Check sheet for the modelled part. Datum: model origin and axes. Units: mm. A direction names the side the tool comes from. Round coordinates to 2 decimals unless told otherwise and drop trailing zeros. Order: outer loops, then holes, each group sorted by start corner. A loop starts at its lowest first (then second) coordinate and runs counter-clockwise, first axis right, second up.
Q1. Mould release check, pull along Z, two halves, no side actions. Record for faces 5 (the flat face through (7, 5, -70)), 6 (the flat face through (118, 20, -120)), 7 (the flat face through (13, 10, -2)): +Z half, -Z half, draft (parallel to the pull), parting line (faces both ways), or undercut.
Q2. Cross-section at D-D on y = 14. Record the cut outline in (x, z), then the cut area to 3 significant figures.
Q3. Scan lines: probe 1 along X at (y, z) = (14, 90); probe 2 along Z at (x, y) = (40, 27.5); probe 3 along Y at (x, z) = (46.5, 36). Record each from-to range of solid material in increasing order.
Q4. Cross-section at B-B on z = 45. Record the cut outline in (x, y), then the cut area to 3 significant figures.
Q5. Depth check by flat-ended pin: P1, Ø8, axis at x = 230.5, z = 47, coming from the +Y side; P2, Ø10, axis at y = 21, z = 48.5, coming from the -X side; P3, Ø5, axis at y = 34.5, z = 90, coming from the +X side. Enter the tip coordinate at first touch or a pass-through.
Q6. Cross-section at C-C on y = 31. Record the cut outline in (x, z), then the cut area to 3 significant figures.
Q7. Cross-section at A-A on x = 78. Record the cut outline in (y, z), then the cut area to 3 significant figures.
Q8. Set-up check for faces 1 (the flat face through (118.687, 32.395, 69.932)), 2 (the flat face through (233, 5, 70)), 3 (the flat face through (227, 10, -2)), 4 (the flat face through (26.245, 22, 2)): record each of +Z, -Z, +X, -X, +Y, -Y from which the full face is reachable in a straight line by a thin tool's end or side.
from build123d import *

# Parameters (mm, degrees)
EXTRUDE_1_DEPTH     = 240
CUT_EXTRUDE_1_DEPTH = 41
SKETCH_3_W          = 26.245299516
SKETCH_3_H          = 240
CUT_EXTRUDE_2_DEPTH = 30


with BuildPart() as part:
    # Эскиз1 → Бобышка-Вытянуть1 (new body)
    with BuildSketch(Plane(origin=(0, 0, 0), x_dir=(0, 0, -1), z_dir=(1, 0, 0))):
        Polygon((-120, 0), (120, 0), (120, 40), (64.71995712, 40), (75, 25), (-75, 25), (-64.71995712, 40), (-120, 40), align=None)
    extrude(amount=EXTRUDE_1_DEPTH)

    # Эскиз2 → Вырез-Вытянуть1 (cut, through all)
    with BuildSketch(Plane.XZ):
        with BuildLine():
            Line((240, 80), (240, 70))
            Line((240, 70), (225, 70))
            ThreePointArc((225, 70), (220, 75), (225, 80))
            Line((225, 80), (240, 80))
        make_face()
        with BuildLine():
            Line((0, -80), (0, -70))
            Line((0, -70), (15, -70))
            ThreePointArc((15, -70), (20, -75), (15, -80))
            Line((15, -80), (0, -80))
        make_face()
    extrude(amount=-CUT_EXTRUDE_1_DEPTH, mode=Mode.SUBTRACT)

    # Эскиз3 → Вырез-Вытянуть2 (cut)
    with BuildSketch(Plane(origin=(0, 40, 0), x_dir=(1, 0, 0), z_dir=(0, 1, 0))):
        with Locations((13.122649758, 0)):
            Rectangle(SKETCH_3_W, SKETCH_3_H)
        with Locations((226.877350242, 0)):
            Rectangle(SKETCH_3_W, SKETCH_3_H)
    extrude(amount=-CUT_EXTRUDE_2_DEPTH, mode=Mode.SUBTRACT)


solid = part.part
Results found:
1. face 5: undercut
1. face 6: -Z half
1. face 7: draft
2. outline: (26.25, -120) - (213.75, -120) - (213.75, 120) - (26.25, 120) - close
2. area: 45,000 mm2
3. probe 1: x = 26.25 to 213.75
3. probe 2: z = -120 to -73.29, 73.29 to 120
3. probe 3: y = 0 to 25
4. outline: (0, 0) - (240, 0) - (240, 10) - (213.75, 10) - (213.75, 25) - (26.25, 25) - (26.25, 10) - (0, 10) - close
4. area: 5,210 mm2
5. P1: stops at y = 10
5. P2: stops at x = 26.25
5. P3: stops at x = 213.75
6. outline: (26.25, -120) - (213.75, -120) - (213.75, -70.89) - (26.25, -70.89) - close; (26.25, 70.89) - (213.75, 70.89) - (213.75, 120) - (26.25, 120) - close
6. area: 18,400 mm2
7. outline: (0, -120) - (40, -120) - (40, -64.72) - (25, -75) - (25, 75) - (40, 64.72) - (40, 120) - (0, 120) - close
7. area: 7,500 mm2
8. face 1: +X, -X
8. face 2: +X, +Y, -Y
8. face 3: +Z, -Z, +X, +Y
8. face 4: +Z, -Z, -X, +Y
